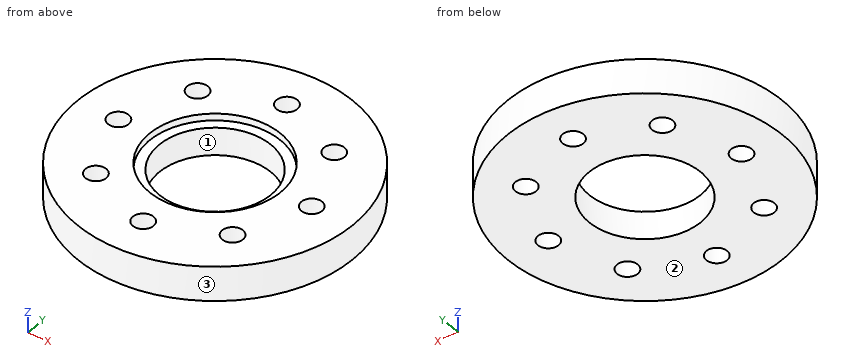
Autodesk Inventor part; units mm, degrees
ref_plane "YZ Plane" through (0, 0, 0) normal (1, 0, 0) x (0, 1, 0)
ref_plane "XZ Plane" through (0, 0, 0) normal (0, 1, 0) x (-1, 0, 0)
ref_plane "XY Plane" through (0, 0, 0) normal (0, 0, 1) x (1, 0, 0)
sketch "スケッチ1" plane through (0, 0, 0) normal (0, 0, 1) x (1, 0, 0)
  circle A0 centre (0, 0) radius 10
  dimension "d0" = 20
extrude "押し出し1" add sketch "スケッチ1" along normal blind 2.5
sketch "スケッチ2" plane through (0, 0, 2.5) normal (0, 0, 1) x (1, 0, 0)
  circle A0 centre (0, 0) radius 10
  circle A1 centre (0, 0) radius 5
  dimension "d3" = 10
hole "穴2" at (0, 0, 2.5) direction (0, 0, -1) diameter 8.1 end through all counterbore diameter 9.5 counterbore depth 0.5
sketch "スケッチ5" plane through (0, 0, 2.5) normal (0, 0, 1) x (1, 0, 0)
  circle A0 centre (0, 7) radius 1
  circle A1 centre (0, 0) radius 4.75
  dimension "d30" = 2
  dimension "d57" = 0
  dimension "d58" = 7
hole "穴4" at (0, 7, 2.5) direction (0, 0, -1) diameter 1.5 end through all
pattern_circular "円形状パターン1" count 8 over 360 about axis through (0, 0, -25.8945) along (0, 0, 1) of "穴4"
properties part number "03" material "アルミニウム 6061"
The listing builds one solid part. Answer for the finished solid, in the listing's coordinates (mm). Face numbers are marked on the shaded views. Round coordinates to 2 decimals unless told otherwise and drop trailing zeros. Write each loop counter-clockwise with the first axis right and the second up, starting at its lowest first coordinate (ties: lowest second). Pieces come first, ordered by that corner, then holes. Notation, with made-up numbers: (85, 53) -> (117, 53) arc R20 cw to (117, 78) -> close; hole circle Ø5 at (50.25, -14.75). An arc over 180 degrees is marked (long way). Answer as a JSON object with one key per item and string values. Group by question number.
Q1. This flat-tipped pin is pushed along its axis until it touches: pin 1 Ø5 at (x, y) = (-2, 0) entering from +Z. Where does it stop, or does it pass through?
Q2. Straight lines are drawn through the part: line 1 along Y through (x, z) = (0.25, 1.25); line 2 along X through (y, z) = (-5.25, 1.8); line 3 along Y through (x, z) = (3, 1.95). For each, find the intervals that lie inside material, in ascending order.
Q3. Determine the mould class of the marked faces 1, 2 and 3 for opening direction X: pulls with the +X half, pulls with the -X half, needs draft (parallel to the pull), parting line crosses it, or undercut.
Q4. Section A-A (x = 7) is taken. Write down the section's boundary in (y, z), plus the area to 3 significant figures.
Q5. Section C-C (z = 2.25) is taken. Count the separate pieces of the cut face and the enclosed holes in it, plus the area to 3 significant figures.
Q6. Section B-B (y = -5.25) is taken. Write down the section's boundary in (x, z).
Q7. Section D-D (y = 1.75) is taken. Write down the section's boundary in (x, z), plus the area to 3 significant figures.
Check values:
{
 "1": {"pin 1": "z = 2"},
 "2": {"line 1": "-10 to -7.71, -6.29 to -4.04, 4.04 to 6.29, 7.71 to 10", "line 2": "-8.51 to -5.64, -4.26 to 4.26, 5.64 to 8.51", "line 3": "-9.54 to -2.72, 2.72 to 9.54"},
 "3": {"face 1": "undercut", "face 2": "needs draft", "face 3": "parting line crosses it"},
 "4": {"outline": "(-7.14, 0) -> (-0.75, 0) -> (-0.75, 2.5) -> (-7.14, 2.5) -> close; (0.75, 0) -> (7.14, 0) -> (7.14, 2.5) -> (0.75, 2.5) -> close", "area": "32.0 mm^2"},
 "5": {"separate pieces": "1", "enclosed holes": "9", "area": "229 mm^2"},
 "6": {"outline": "(-8.51, 0) -> (-5.64, 0) -> (-5.64, 2.5) -> (-8.51, 2.5) -> close; (-4.26, 0) -> (4.26, 0) -> (4.26, 2.5) -> (-4.26, 2.5) -> close; (5.64, 0) -> (8.51, 0) -> (8.51, 2.5) -> (5.64, 2.5) -> close"},
 "7": {"outline": "(-9.85, 0) -> (-3.65, 0) -> (-3.65, 2) -> (-4.42, 2) -> (-4.42, 2.5) -> (-9.85, 2.5) -> close; (3.65, 0) -> (9.85, 0) -> (9.85, 2.5) -> (4.42, 2.5) -> (4.42, 2) -> (3.65, 2) -> close", "area": "30.2 mm^2"}
}
